Verification items for the finished model (mm, model axes). Face numbers are marked on the shaded views. Give positions to 0.01 mm unless a question says otherwise; leave off trailing zeros. Order: outer loops, then holes, each group sorted by start corner. A loop starts at its lowest first (then second) coordinate and runs counter-clockwise, first axis right, second up. Notation, with made-up numbers: (48.5, 5.5) -> (70.5, 5.5) arc R33 ccw to (70.5, 37.5) -> close; hole circle Ø2 at (48, 58). An arc over 180 degrees is marked (long way). Write each question's results on one line, items separated by ' | '. Start each with the question number.
1. Cross-section at C-C, the plane x = -686.5. Enter the section's corners in (y, z), then the cut area to 3 significant figures.
2. Mould release check, pull along X, two halves, no side actions. Record for the marked faces 1 and 2: +X half, -X half, draft (parallel to the pull), parting line (faces both ways), or undercut.
3. Material ranges on L1, parallel to Z at x = -476.25, y = -0.95; L2, parallel to X at y = -1, z = -19; L3, parallel to X at y = -2, z = -19, recorded low to high. Write a range as from..to.
4. Depth check by flat-ended pin: pin 1 Ø3 at (y, z) = (-122, -80.5) entering from +X; pin 2 Ø10 at (x, z) = (-807, -125) entering from -Y; pin 3 Ø5 at (y, z) = (-217.5, -100) entering from +X. Enter the tip coordinate at first touch or a pass-through.
5. Cross-section at A-A, the plane z = -102.5. Enter the section's corners in (x, y).
6. Cross-section at B-B, the plane y = -51. Enter the section's corners in (x, z), then the cut area to 3 significant figures.
7. Cross-section at D-D, the plane x = -328. Enter the section's corners in (y, z).
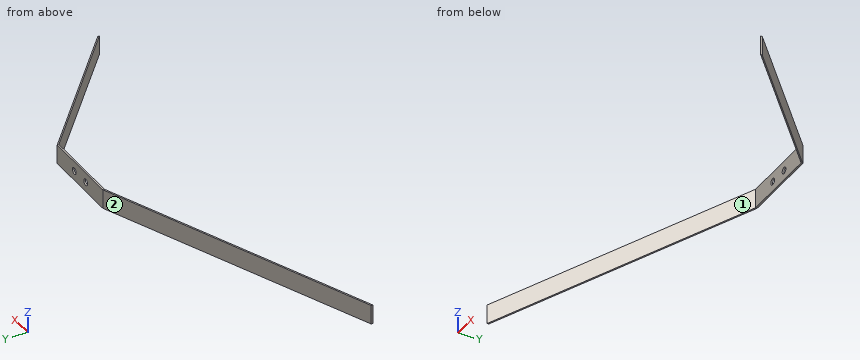
from build123d import *

# Parameters (mm, degrees)
F0_W      = 914.4
F0_H      = 152.4
F1_DEPTH  = 304.8
F3_DEPTH  = 152.401
F5_DEPTH  = 152.401
F7_DEPTH  = 152.401
F9_DEPTH  = 304.801
F11_DEPTH = 304.801
F13_DEPTH = 304.801
F15_D     = 12.7


with BuildPart() as f1:
    # F0 (on Front) → F1 (new body)
    with BuildSketch(Plane.XZ):
        with Locations((-457.2, -76.2)):
            Rectangle(F0_W, F0_H)
    extrude(amount=F1_DEPTH)

    # F2 (on face) → F3 (cut, through all)
    with BuildSketch(Plane.XY):
        Polygon((-381, -3.175), (-533.4, -3.175), (-914.4, -304.8), (0, -304.8), align=None)
    extrude(amount=-F3_DEPTH, mode=Mode.SUBTRACT)

    # F4 (on face) → F5 (cut, through all)
    with BuildSketch(Plane.XY):
        Polygon((-914.4, 0), (-914.4, -301.625), (-533.4, 0), align=None)
    extrude(amount=-F5_DEPTH, mode=Mode.SUBTRACT)

    # F6 (on face) → F7 (cut, through all)
    with BuildSketch(Plane.XY):
        Polygon((0, 0), (-381, 0), (0, -301.625), align=None)
    extrude(amount=-F7_DEPTH, mode=Mode.SUBTRACT)

    # F8 (on face) → F9 (cut, through all)
    with BuildSketch(Plane(origin=(0, 0, 0), x_dir=(-1, 0, 0), z_dir=(0, 1, 0))):
        Polygon((381, -38.1), (0, -152.4), (914.4, -152.4), (533.4, -38.1), align=None)
    extrude(amount=-F9_DEPTH, mode=Mode.SUBTRACT)

    # F10 (on face) → F11 (cut, through all)
    with BuildSketch(Plane(origin=(0, 0, 0), x_dir=(-1, 0, 0), z_dir=(0, 1, 0))):
        Polygon((0, -114.3), (381, 0), (0, 0), align=None)
    extrude(amount=-F11_DEPTH, mode=Mode.SUBTRACT)

    # F12 (on face) → F13 (cut, through all)
    with BuildSketch(Plane(origin=(0, 0, 0), x_dir=(-1, 0, 0), z_dir=(0, 1, 0))):
        Polygon((914.4, 0), (533.4, 0), (914.4, -114.3), align=None)
    extrude(amount=-F13_DEPTH, mode=Mode.SUBTRACT)

    # F15 (through all)
    with Locations(Plane.XZ.offset(3.175)):
        with Locations((-476.25, -19.05), (-438.15, -19.05)):
            Hole(F15_D / 2)


solid = f1.part
Results below:
1) outline: (-124.38, -84.03) -> (-121.2, -84.03) -> (-121.2, -45.93) -> (-124.38, -45.93) -> close | area: 121 mm²
2) face 1: undercut | face 2: -X half
3) L1: z = -38.1..-25.4, -12.7..0 | L2: x = -534.66..-482.6, -469.9..-444.5, -431.8..-379.74 | L3: x = -535.93..-482.6, -469.9..-444.5, -431.8..-378.47
4) pin 1: stops at x = -225 | pin 2: stops at y = -222.28 | pin 3: stops at x = -103.11
5) outline: (-875.07, -273.66) -> (-748.07, -173.12) -> (-748.07, -169.94) -> (-875.07, -270.49) -> close; (-166.33, -173.12) -> (-39.33, -273.66) -> (-39.33, -270.49) -> (-166.33, -169.94) -> close
6) outline: (-597.82, -57.43) -> (-593.81, -56.22) -> (-593.81, -18.12) -> (-597.82, -19.33) -> close; (-320.59, -56.22) -> (-316.58, -57.43) -> (-316.58, -19.33) -> (-320.59, -18.12) -> close | area: 306 mm²
7) outline: (-45.13, -54) -> (-41.96, -54) -> (-41.96, -15.9) -> (-45.13, -15.9) -> close
